from build123d import *

# Parameters (mm, degrees)
BOSS_EXTRUDE1_DEPTH = 304.8
SKETCH2_R           = 14.2875
CUT_EXTRUDE1_DEPTH  = 304.8
FILLET1_R           = 25.4
FILLET2_R           = 25.4


with BuildPart() as part:
    # Sketch1 → Boss-Extrude1 (new body)
    with BuildSketch(Plane.XY):
        Polygon((0, 0), (-63.5, 25.4), (-63.5, 107.589933746), (-15.875, 132.989933746), (-15.875, 183.789933746), (-22.225, 183.789933746), (-22.225, 136.799933746), (-69.85, 111.399933746), (-69.85, 21.100840695), (0, -6.839159305), (69.85, 21.100840695), (69.85, 111.399933746), (22.225, 136.799933746), (22.225, 183.789933746), (15.875, 183.789933746), (15.875, 132.989933746), (63.5, 107.589933746), (63.5, 25.4), align=None)
    extrude(amount=BOSS_EXTRUDE1_DEPTH)

    # Sketch2 → Cut-Extrude1 (cut)
    with BuildSketch(Plane(origin=(22.225, 0, 0), x_dir=(0, 0, -1), z_dir=(1, 0, 0))):
        with Locations((-266.7, 160.294933746)):
            Circle(SKETCH2_R)
        Polygon((-17.921004613, 160.294933746), (-21.660502306, 166.771933746), (-29.139497694, 166.771933746), (-32.878995387, 160.294933746), (-29.139497694, 153.817933746), (-21.660502306, 153.817933746), align=None)
    extrude(amount=-CUT_EXTRUDE1_DEPTH, mode=Mode.SUBTRACT)

    # Fillet1
    fillet1_edges = [part.edges().sort_by_distance(p)[0] for p in [
        (19.05, 183.789933746, 0),
        (-19.05, 183.789933746, 0),
    ]]
    fillet(fillet1_edges, radius=FILLET1_R)

    # Fillet2
    fillet2_edges = [part.edges().sort_by_distance(p)[0] for p in [
        (-19.05, 183.789933746, 304.8),
        (19.05, 183.789933746, 304.8),
    ]]
    fillet(fillet2_edges, radius=FILLET2_R)


solid = part.part
Input: part model. Units: mm. Frame: model coordinates. A direction names the side the tool comes from. Give positions to 0.01 mm unless a question says otherwise; leave off trailing zeros. Loops run counter-clockwise (first coordinate to the right, second up) from the corner with the lowest first, then second, coordinate; pieces in that order, holes last. Notation, with made-up numbers: (15.25, -30.5) - (69.25, -30.5) arc R22 ccw to (69.25, -11.5) - close; hole circle Ø3 at (35.5, 12). An arc over 180 degrees is marked (long way). Use CSV: the item, a comma, the result in double quotes. Start each with the question number.
Item 1: Reachability of faces 5 (the flat face through (15.875, 159, 150)), 6 (the flat face through (22.225, 160, 150)), 7 (the flat face through (-31.4, 125.1, 0)), 8 (the flat face through (-19.006, 157.102, 31.035)), 9 (the flat face through (32.194, 12.878, 150.266)) from +Z, -Z, +X, -X, +Y, -Y: full face, straight path, thin tool, end or side. Return the list, or none.
Item 2: Section C-C on x = -44.5. Return loops of the section in (y, z).
Item 3: Section A-A on z = 266.7. Return loops of the section in (x, y) (3 decimals), then the cut area to 3 significant figures.
Item 4: Section B-B on y = 61. Return loops of the section in (x, z).
Item 5: Section D-D on z = 94. Return loops of the section in (x, y) (3 decimals).
Item 6: Line query: line 1 (X direction, y = 40.5, z = 285); line 2 (Y direction, x = -21, z = 266.7); line 3 (Y direction, x = 62, z = 166.5). Output: solid intervals per line, ascending.
Item 7: Contact query for flat-ended pins moving along their axis: P1, Ø3, axis at x = -18.5, z = 25.5, coming from the -Y side; P2, Ø4, axis at x = 6.5, z = 129, coming from the -Y side; P3, Ø4, axis at y = 14.5, z = 45, coming from the -X side. Output: stop coordinate, or through.
Item 8: Mould query, pull axis Y, two halves, no side actions, for faces 1 (the flat face through (-69.85, 67, 150)), 2 (the flat face through (-45.7, 124.28, 150.27)), 3 (the flat face through (63.5, 67, 150)), 4 (the flat face through (19, 153.818, 25)). Classes: pulls with the +Y half, pulls with the -Y half, needs draft (parallel to the pull), parting line crosses it, or undercut.
Ans:
1,face 5,"+Z, -Z, +Y"
1,face 6,"+Z, -Z, +X, +Y"
1,face 7,"-Z, +X, -X, +Y, -Y"
1,face 8,"+X, -X"
1,face 9,"+Z, -Z"
2,outline,"(10.96, 0) - (17.8, 0) - (17.8, 304.8) - (10.96, 304.8) - close; (117.72, 0) - (124.92, 0) - (124.92, 304.8) - (117.72, 304.8) - close"
3,outline,"(-69.85, 21.101) - (0, -6.839) - (69.85, 21.101) - (69.85, 111.4) - (22.225, 136.8) - (22.225, 146.007) - (15.875, 146.007) - (15.875, 132.99) - (63.5, 107.59) - (63.5, 25.4) - (0, 0) - (-63.5, 25.4) - (-63.5, 107.59) - (-15.875, 132.99) - (-15.875, 146.007) - (-22.225, 146.007) - (-22.225, 136.8) - (-69.85, 111.4) - close; (-22.225, 174.582) - (-15.875, 174.582) - (-15.875, 183.79) - (-22.225, 183.79) - close; (15.875, 174.582) - (22.225, 174.582) - (22.225, 183.79) - (15.875, 183.79) - close"
3,area,"2,950 mm2"
4,outline,"(-69.85, 0) - (-63.5, 0) - (-63.5, 304.8) - (-69.85, 304.8) - close; (63.5, 0) - (69.85, 0) - (69.85, 304.8) - (63.5, 304.8) - close"
5,outline,"(-69.85, 21.101) - (0, -6.839) - (69.85, 21.101) - (69.85, 111.4) - (22.225, 136.8) - (22.225, 183.79) - (15.875, 183.79) - (15.875, 132.99) - (63.5, 107.59) - (63.5, 25.4) - (0, 0) - (-63.5, 25.4) - (-63.5, 107.59) - (-15.875, 132.99) - (-15.875, 183.79) - (-22.225, 183.79) - (-22.225, 136.8) - (-69.85, 111.4) - close"
6,line 1,"x = -69.85 to -63.5, 63.5 to 69.85"
6,line 2,"y = 1.56 to 8.4, 130.26 to 146.01, 174.58 to 183.79"
6,line 3,"y = 17.96 to 24.8, 108.39 to 115.59"
7,P1,"stops at y = -0.04"
7,P2,"stops at y = -5.04"
7,P3,"stops at x = -58.35"
8,face 1,"needs draft"
8,face 2,"pulls with the +Y half"
8,face 3,"undercut"
8,face 4,"undercut"
